Answer from the drawing. Dimensions are ordinates in mm from the lowest x, y and z of the part. A direction names the side the tool comes from. Coordinates: 2 decimals unless noted, no trailing zeros. Write each loop counter-clockwise with the first axis right and the second up, starting at its lowest first coordinate (ties: lowest second). Pieces come first, ordered by that corner, then holes.
(1) For a pull along Z with two mould halves and no side action, classify the marked faces 1, 2, 3 and 4 as +Z half, -Z half, draft (parallel to the pull), parting line (faces both ways), or undercut.
(2) The part is cut by section B-B on z = 19.5. Determine the outline of the cut face in (x, y).
(3) The part is cut by section D-D on z = 61.5. Determine the outline of the cut face in (x, y).
(4) The part is cut by section A-A on y = 279.5. Determine the outline of the cut face in (x, z).
(5) Given P1, Ø3, axis at y = 192, z = 77, coming from the -X side; P2, Ø10, axis at x = 61.5, z = 43, coming from the +Y side, each flat-ended and moving along its own axis, determine where each tip first touches the part or whether it passes through.
(6) The part is cut by section C-C on x = 19.5. Determine the outline of the cut face in (y, z).
(7) Which of the six approach directions +Z, -Z, +X, -X, +Y, -Y give full straight-line access (tool end or side, diameter ignored) to the marked faces 5 and 6?
(8) Straight lines are drawn through the part: line 1 (X direction, y = 259.5, z = 85.5); line 2 (Y direction, x = 31.5, z = 5.5). For each, find the intervals that lie inside material, in ascending order.
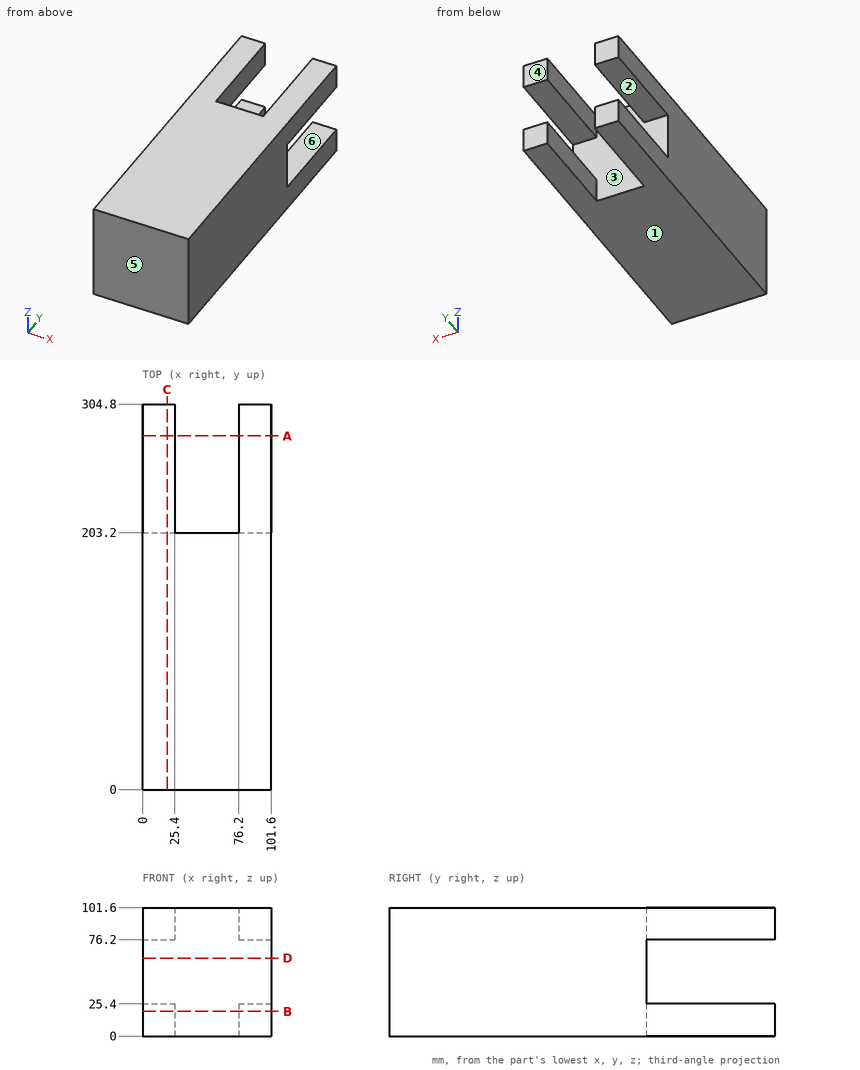
Model answer:
1. face 1: -Z half
1. face 2: undercut
1. face 3: undercut
1. face 4: draft
2. outline: (0, 0) - (101.6, 0) - (101.6, 304.8) - (76.2, 304.8) - (76.2, 203.2) - (25.4, 203.2) - (25.4, 304.8) - (0, 304.8) - close
3. outline: (0, 0) - (101.6, 0) - (101.6, 203.2) - (0, 203.2) - close
4. outline: (0, 0) - (25.4, 0) - (25.4, 25.4) - (0, 25.4) - close; (0, 76.2) - (25.4, 76.2) - (25.4, 101.6) - (0, 101.6) - close; (76.2, 0) - (101.6, 0) - (101.6, 25.4) - (76.2, 25.4) - close; (76.2, 76.2) - (101.6, 76.2) - (101.6, 101.6) - (76.2, 101.6) - close
5. P1: stops at x = 0
5. P2: stops at y = 203.2
6. outline: (0, 0) - (304.8, 0) - (304.8, 25.4) - (203.2, 25.4) - (203.2, 76.2) - (304.8, 76.2) - (304.8, 101.6) - (0, 101.6) - close
7. face 5: +Z, -Z, +X, -X, -Y
7. face 6: +X, -X, +Y
8. line 1: x = 0 to 25.4, 76.2 to 101.6
8. line 2: y = 0 to 203.2
